```python
from build123d import *

# Parameters (mm, degrees)
SKETCH1_R           = 12.7
BOSS_EXTRUDE1_DEPTH = 5.842
SKETCH2_R           = 0.1984375
CUT_EXTRUDE1_DEPTH  = 19.886740428


with BuildPart() as part:
    # Sketch1 → Boss-Extrude1 (new body)
    with BuildSketch(Plane.XY):
        Circle(SKETCH1_R)
        Polygon((-7.274613392, 0), (-3.637306696, -6.3), (3.637306696, -6.3), (7.274613392, 0), (3.637306696, 6.3), (-3.637306696, 6.3), align=None, mode=Mode.SUBTRACT)
    extrude(amount=BOSS_EXTRUDE1_DEPTH)

    # Sketch2 → Cut-Extrude1 (cut, through all)
    with BuildSketch(Plane.XY.offset(5.842)):
        with Locations((3.637306696, 6.3)):
            Circle(SKETCH2_R)
        with Locations((-3.637306696, 6.3)):
            Circle(SKETCH2_R)
        with Locations((-7.274613392, 0)):
            Circle(SKETCH2_R)
        with Locations((-3.637306696, -6.3)):
            Circle(SKETCH2_R)
        with Locations((3.637306696, -6.3)):
            Circle(SKETCH2_R)
        with Locations((7.274613392, 0)):
            Circle(SKETCH2_R)
    extrude(amount=-CUT_EXTRUDE1_DEPTH, mode=Mode.SUBTRACT)


solid = part.part
```
Read the model definition and answer for the solid it produces. Units are mm, in the model's axes. A direction names the side the tool comes from. Coordinates: 2 decimals unless noted, no trailing zeros. Write each loop counter-clockwise with the first axis right and the second up, starting at its lowest first coordinate (ties: lowest second). Pieces come first, ordered by that corner, then holes. Notation, with made-up numbers: (-36, -28) - (22, -28) arc R15 cw to (22, -23) - close; hole circle Ø6 at (40.5, -38.5). An arc over 180 degrees is marked (long way). Answer as a JSON object with one key per item and string values. Group by question number.
1. This flat-tipped pin is pushed along its axis until it touches: P1, Ø1.5, axis at x = -5, z = 4, coming from the +Y side. Where does it stop, or does it pass through?
2. The mould has two halves that part along X. Classify faces 1 (the flat face through (-6, -3, 0)), 2 (the flat face through (-5.48, -3.11, 2.88)), 3 (the cylindrical face through (-2.75, -12.4, 2.88)): +X half, -X half, draft (parallel to the pull), parting line (faces both ways), or undercut.
3. A cutting plane is placed at A-A (z = 1.1). Determine the outline of the cut face in (x, y).
4. Consider L1, parallel to X at y = 3, z = 4.2; L2, parallel to Y at x = 6, z = 4.95; L3, parallel to Y at x = 4.5, z = 2.65. Determine where each line is inside the solid, lowest interval first. Write a range as [from, to].
5. A cutting plane is placed at B-B (x = 0). Determine the outline of the cut face in (y, z), plus the area to 3 significant figures.
6. A cutting plane is placed at D-D (x = -9). Determine the outline of the cut face in (y, z), plus the area to 3 significant figures.
7. Which of the six approach directions +Z, -Z, +X, -X, +Y, -Y give full straight-line access (tool end or side, diameter ignored) to faces 4 (the flat face through (-6, -3, 5.842)), 5 (the flat face through (5.48, 3.11, 2.88))?
8. A cutting plane is placed at C-C (y = -1.75). Determine the outline of the cut face in (x, z), plus the area to 3 significant figures.
Worked out:
{
 "1": {"P1": "stops at y = 11.97"},
 "2": {"face 1": "draft", "face 2": "undercut", "face 3": "parting line"},
 "3": {"outline": "circle Ø25.4 at (0, 0); hole (-7.18, -0.17) - (-3.74, -6.13) arc R0.2 ccw (long way) to (-3.44, -6.3) - (3.44, -6.3) arc R0.2 ccw (long way) to (3.74, -6.13) - (7.18, -0.17) arc R0.2 ccw (long way) to (7.18, 0.17) - (3.74, 6.13) arc R0.2 ccw (long way) to (3.44, 6.3) - (-3.44, 6.3) arc R0.2 ccw (long way) to (-3.74, 6.13) - (-7.18, 0.17) arc R0.2 ccw (long way) to start"},
 "4": {"L1": "x = [-12.34, -5.54], [5.54, 12.34]", "L2": "y = [-11.19, -2.21], [2.21, 11.19]", "L3": "y = [-11.88, -4.81], [4.81, 11.88]"},
 "5": {"outline": "(-12.7, 0) - (-6.3, 0) - (-6.3, 5.84) - (-12.7, 5.84) - close; (6.3, 0) - (12.7, 0) - (12.7, 5.84) - (6.3, 5.84) - close", "area": "74.8 mm²"},
 "6": {"outline": "(-8.96, 0) - (8.96, 0) - (8.96, 5.84) - (-8.96, 5.84) - close", "area": "105 mm²"},
 "7": {"face 4": "+Z, +X, -X, +Y, -Y", "face 5": "+Z, -Z"},
 "8": {"outline": "(-12.58, 0) - (-6.26, 0) - (-6.26, 5.84) - (-12.58, 5.84) - close; (6.26, 0) - (12.58, 0) - (12.58, 5.84) - (6.26, 5.84) - close", "area": "73.8 mm²"}
}
